The model under review builds one solid part; all positions refer to its coordinate system, in mm. A direction names the side the tool comes from. Coordinates: 2 decimals unless noted, no trailing zeros. Write each loop counter-clockwise with the first axis right and the second up, starting at its lowest first coordinate (ties: lowest second). Pieces come first, ordered by that corner, then holes. Notation, with made-up numbers: (73, 16.5) - (122, 16.5) arc R21 ccw to (122, 28.5) - close; hole circle Ø4 at (46, 44.25). An arc over 180 degrees is marked (long way). Put each result on its own line as item: value.
from build123d import *

# Parameters (mm, degrees)
Y_KSEKLIK_EKSTR_ZYON1_DEPTH             = 6
M3X0_5_HELISARMAL_IN_DI_LI_DELIK1_D     = 3.15
M3X0_5_HELISARMAL_IN_DI_LI_DELIK1_DEPTH = 7.5
M3X0_5_HELISARMAL_IN_DI_LI_DELIK1_TIP   = 0.946355475
M8X1_0_HELISARMAL_IN_DI_LI_DELIK2_D     = 8.25
M8X1_0_HELISARMAL_IN_DI_LI_DELIK2_DEPTH = 18
M8X1_0_HELISARMAL_IN_DI_LI_DELIK2_TIP   = 2.478550053
IZIM7_R                                 = 6.5
KES_EKSTR_ZYON1_DEPTH                   = 10


with BuildPart() as part:
    # Çizim1 → Yükseklik-Ekstrüzyon1 (new body)
    with BuildSketch(Plane.XY):
        with BuildLine():
            Line((32.040014045, 45), (24, 45))
            Line((24, 45), (24, 21.6))
            Line((24, 21.6), (-24, 21.6))
            Line((-24, 21.6), (-24, 45))
            Line((-24, 45), (-32.040014045, 45))
            ThreePointArc((-32.040014045, 45), (-33.696486936, 44.717636862), (-35.165869074, 43.902439024))
            ThreePointArc((-35.165869074, 43.902439024), (-56.25, 0), (-35.165869074, -43.902439024))
            ThreePointArc((-35.165869074, -43.902439024), (-33.696486936, -44.717636862), (-32.040014045, -45))
            Line((-32.040014045, -45), (32.040014045, -45))
            ThreePointArc((32.040014045, -45), (33.696486936, -44.717636862), (35.165869074, -43.902439024))
            ThreePointArc((35.165869074, -43.902439024), (56.25, 0), (35.165869074, 43.902439024))
            ThreePointArc((35.165869074, 43.902439024), (33.696486936, 44.717636862), (32.040014045, 45))
        make_face()
    extrude(amount=Y_KSEKLIK_EKSTR_ZYON1_DEPTH)

    # M3x0.5 Helisarmal İçin Dişli Delik1
    with Locations(Plane(origin=(0, 0, 0), x_dir=(-1, 0, 0), z_dir=(0, 0, -1))):
        with Locations((38.338421514, -35.130690796), (52, 0), (-52, 0), (-36.769552622, 36.769552622), (-45.033320997, -26), (36.769552622, 36.769552622), (45.033320997, -26), (-38.338421514, -35.130690796)):
            Hole(M3X0_5_HELISARMAL_IN_DI_LI_DELIK1_D / 2, depth=M3X0_5_HELISARMAL_IN_DI_LI_DELIK1_DEPTH)
            with Locations((0, 0, -(M3X0_5_HELISARMAL_IN_DI_LI_DELIK1_DEPTH + M3X0_5_HELISARMAL_IN_DI_LI_DELIK1_TIP / 2))):  # 118° drill point
                Cone(0, M3X0_5_HELISARMAL_IN_DI_LI_DELIK1_D / 2, M3X0_5_HELISARMAL_IN_DI_LI_DELIK1_TIP, mode=Mode.SUBTRACT)

    # M8x1.0 Helisarmal İçin Dişli Delik2
    with Locations(Plane(origin=(0, 0, 0), x_dir=(-1, 0, 0), z_dir=(0, 0, -1))):
        with Locations((-31.720772546, 14.791639161)):
            Hole(M8X1_0_HELISARMAL_IN_DI_LI_DELIK2_D / 2, depth=M8X1_0_HELISARMAL_IN_DI_LI_DELIK2_DEPTH)
            with Locations((0, 0, -(M8X1_0_HELISARMAL_IN_DI_LI_DELIK2_DEPTH + M8X1_0_HELISARMAL_IN_DI_LI_DELIK2_TIP / 2))):  # 118° drill point
                Cone(0, M8X1_0_HELISARMAL_IN_DI_LI_DELIK2_D / 2, M8X1_0_HELISARMAL_IN_DI_LI_DELIK2_TIP, mode=Mode.SUBTRACT)

    # Çizim7 → Kes-Ekstrüzyon1 (cut)
    with BuildSketch(Plane(origin=(0, 0, 0), x_dir=(-1, 0, 0), z_dir=(0, 0, -1))):
        with Locations((31.720772546, -14.791639161)):
            Circle(IZIM7_R)
    extrude(amount=-KES_EKSTR_ZYON1_DEPTH, mode=Mode.SUBTRACT)


solid = part.part
1. Consider section B-B on x = -52. State the section outline as (y, z) points (3 decimals), plus the area to 3 significant figures.
Determined:
outline: (-21.449, 0) - (-1.575, 0) - (-1.575, 6) - (-21.449, 6) - close; (1.575, 0) - (21.449, 0) - (21.449, 6) - (1.575, 6) - close
area: 238 mm^2
2. Machinability: for faces 4 (the flat face through (-24, 33, 3)), 5 (the flat face through (-28, 45, 3)), which of the approach directions +Z, -Z, +X, -X, +Y, -Y give a long, thin tool a straight path to every point of the face, cutting with its end or side? Answer none if there is none.
Determined:
face 4: +Z, -Z, +Y
face 5: +Z, -Z, +X, -X, +Y
3. Consider section D-D on z = 2.4. Give the number of separate pieces and of enclosed holes in the cut face, plus the area to 3 significant figures.
Determined:
separate pieces: 1
enclosed holes: 10
area: 7,530 mm^2
4. For pin 1 Ø1.9 at (x, y) = (-45.03, -26) entering from +Z; pin 2 Ø1.8 at (y, z) = (33, 4.5) entering from +X; pin 3 Ø1.8 at (x, z) = (5, 3) entering from +Y; pin 4 Ø5 at (x, y) = (-38.34, -35.13) entering from +Z, all flat-tipped, find the tip position at first contact; note any pin that passes through.
Determined:
pin 1: passes through
pin 2: stops at x = 46.19
pin 3: stops at y = 21.6
pin 4: stops at z = 6
5. Consider section C-C on y = -11. State the section outline as (x, z) points.
Determined:
outline: (-55.16, 0) - (-37, 0) - (-37, 6) - (-55.16, 6) - close; (-26.44, 0) - (55.16, 0) - (55.16, 6) - (-26.44, 6) - close
6. The part is to be moulded in two halves that separate along Y. For faces 1 (the flat face through (24, 33, 3)), 2 (the flat face through (0, 21.6, 3)), 3 (the cylindrical face through (-37.492, -33.803, 3.042)), say which applies: +Y half, -Y half, draft (parallel to the pull), parting line (faces both ways), or undercut.
Determined:
face 1: draft
face 2: +Y half
face 3: undercut
7. Consider section A-A on y = 0. State the section outline as (x, z) points (3 decimals), plus the area to 3 significant figures.
Determined:
outline: (-56.25, 0) - (-53.575, 0) - (-53.575, 6) - (-56.25, 6) - close; (-50.425, 0) - (50.425, 0) - (50.425, 6) - (-50.425, 6) - close; (53.575, 0) - (56.25, 0) - (56.25, 6) - (53.575, 6) - close
area: 637 mm^2
8. To check wall thickness, follow probe 1 along X at (y, z) = (38, 0.7); probe 2 along Y at (x, z) = (-22, 3.25); probe 3 along X at (y, z) = (31.5, 3.5). State the ranges of each line that lie inside material, in increasing order.
Determined:
probe 1: x = -41.47 to -37.75, -35.79 to -24, 24 to 35.79, 37.75 to 41.47
probe 2: y = -45 to 21.6
probe 3: x = -46.6 to -24, 24 to 46.6
